Build history of the part. All positions in model axes, mm. Give positions to 0.01 mm unless a question says otherwise; leave off trailing zeros. Write each loop counter-clockwise with the first axis right and the second up, starting at its lowest first coordinate (ties: lowest second). Pieces come first, ordered by that corner, then holes.
from build123d import *

# Parameters (mm, degrees)
SKETCH1_R           = 4
BOSS_EXTRUDE1_DEPTH = 366
SKETCH2_R           = 1
CUT_EXTRUDE1_DEPTH  = 10
CHAMFER1_SIZE       = 0.5


with BuildPart() as part:
    # Sketch1 → Boss-Extrude1 (new body)
    with BuildSketch(Plane.XY):
        Circle(SKETCH1_R)
    extrude(amount=BOSS_EXTRUDE1_DEPTH)

    # Sketch2 → Cut-Extrude1 (cut)
    with BuildSketch(Plane.XY.offset(366)):
        Circle(SKETCH2_R)
    extrude(amount=-CUT_EXTRUDE1_DEPTH, mode=Mode.SUBTRACT)

    # Chamfer1
    chamfer1_edges = [part.edges().sort_by_distance(p)[0] for p in [
        (-4, 0, 0),
        (-4, 0, 366),
    ]]
    chamfer(chamfer1_edges, length=CHAMFER1_SIZE)


solid = part.part
1. Drill centre lines: line 1 along Y through (x, z) = (0, 360.25); line 2 along Y through (x, z) = (-0.75, 137.5); line 3 along X through (y, z) = (0.25, 234.5). Where is each one in solid material? Low to high.
2. Drop flat-ended pins along their axis: pin 1 (3 mm diameter, centred on x = 0.5, z = 80, fed in from +Y); pin 2 (3 mm diameter, centred on x = -3, z = 204, fed in from -Y); pin 3 (1 mm diameter, centred on x = -2.5, z = 278, fed in from +Y); pin 4 (1.2 mm diameter, centred on x = 0, y = 0, fed in from +Z). Give the stop position or say it passes through.
3. Saw through at A-A on z = 179. Give the cut face in (x, y).
Outcome:
1. line 1: y = -4 to -1, 1 to 4
1. line 2: y = -3.93 to 3.93
1. line 3: x = -3.99 to 3.99
2. pin 1: stops at y = 4
2. pin 2: stops at y = -3.71
2. pin 3: stops at y = 3.46
2. pin 4: stops at z = 356
3. outline: circle Ø8 at (0, 0)
